Can you work these out from the model? Positions are in its coordinate system, mm. Give positions to 0.01 mm unless a question says otherwise; leave off trailing zeros. Order: outer loops, then holes, each group sorted by start corner. A loop starts at its lowest first (then second) coordinate and runs counter-clockwise, first axis right, second up. Notation, with made-up numbers: (0, 9.5) - (56, 9.5) arc R24 ccw to (56, 29.5) - close; hole circle Ø8 at (-24, -14.75). An arc over 180 degrees is marked (long way). Use one line per item in the form item = value. Start each with the question number.
1) Suppose I cut it at D-D, the plane z = -6. Write out the boundary of the cut face in (x, y), and give its area (3 significant figures).
2) For pin 1 (1.5 mm diameter, centred on x = 0.5, z = -2.5, fed in from +Y), with a flat end and sliding along its axis, tell me the tip position at first contact or that it passes through.
3) Suppose I cut it at C-C, the plane y = 0.2. Write out the boundary of the cut face in (x, z), and give its area (3 significant figures).
4) We'd pull the mould along X, two halves only. Please class faces 1 (the flat face through (0, 0.787, -3)), 2 (the flat face through (0, 0.66, -4.7)), 3 (the flat face through (-3.5, 0.4, -6.9)), 4 (the flat face through (3.5, 0.4, -6.9)): released by +X, released by -X, zero draft, split by the parting line, or undercut.
5) Please list where these lines run through material, in increasing order: probe 1 along X at (y, z) = (0.75, -5.25); probe 2 along Y at (x, z) = (-1.75, -2); probe 3 along Z at (x, y) = (0.75, 0.7).
6) Suppose I cut it at B-B, the plane z = -14.5. Write out the boundary of the cut face in (x, y), and give its area (3 significant figures).
```python
from build123d import *

# Parameters (mm, degrees)
SKETCH1_W           = 7
SKETCH1_H           = 11.4
BOSS_EXTRUDE1_DEPTH = 0.6604
BOSS_EXTRUDE2_DEPTH = 7
SKETCH4_R           = 1.07
SKETCH4_W           = 0.625641059
SKETCH4_H           = 1.254110087
BOSS_EXTRUDE3_DEPTH = 0.127
SKETCH5_R           = 0.1
BOSS_EXTRUDE4_DEPTH = 10


with BuildPart() as part:
    # Sketch1 → Boss-Extrude1 (new body)
    with BuildSketch(Plane(origin=(0, 0, 0), x_dir=(1, 0, 0), z_dir=(0, 1, 0))):
        with Locations((0, 5.7)):
            Rectangle(SKETCH1_W, SKETCH1_H)
    extrude(amount=BOSS_EXTRUDE1_DEPTH)

    # Sketch3 → Boss-Extrude2 (add)
    with BuildSketch(Plane.ZY.offset(3.5)):
        with BuildLine():
            Line((-11.4, 0.6604), (-11.4, 1.2))
            ThreePointArc((-11.4, 1.2), (-10.260013654, 1.483539887), (-9.25, 0.883676442))
            Line((-9.25, 0.883676442), (-9.25, 0.6604))
            Line((-9.25, 0.6604), (-11.4, 0.6604))
        make_face()
    extrude(amount=-BOSS_EXTRUDE2_DEPTH)

    # Sketch4 → Boss-Extrude3 (add)
    with BuildSketch(Plane(origin=(0, 0.6604, 0), x_dir=(1, 0, 0), z_dir=(0, 1, 0))):
        with Locations(Location((0, 3.4, 0), (0, 0, 270))):
            Circle(SKETCH4_R)
        with Locations((0.312820529, 5.772944956)):
            Rectangle(SKETCH4_W, SKETCH4_H)
        with BuildLine():
            Line((-0.625641059, 4.901538541), (-0.691025641, 5.058461538))
            ThreePointArc((-0.691025641, 5.058461538), (0, 1.603333333), (0.691025641, 5.058461538))
            Line((0.691025641, 5.058461538), (0.625641059, 4.901538541))
            ThreePointArc((0.625641059, 4.901538541), (0, 1.773333247), (-0.625641059, 4.901538541))
        make_face()
        with BuildLine():
            Line((0.905128238, 5.572307772), (0.970512821, 5.729230769))
            ThreePointArc((0.970512821, 5.729230769), (0, 0.876666667), (-0.970512821, 5.729230769))
            Line((-0.970512821, 5.729230769), (-0.905128238, 5.572307772))
            ThreePointArc((-0.905128238, 5.572307772), (0, 1.046666581), (0.905128238, 5.572307772))
        make_face()
        with BuildLine():
            Line((1.184615418, 6.243077002), (1.25, 6.4))
            ThreePointArc((1.25, 6.4), (0, 0.15), (-1.25, 6.4))
            Line((-1.25, 6.4), (-1.184615418, 6.243077002))
            ThreePointArc((-1.184615418, 6.243077002), (0, 0.319999914), (1.184615418, 6.243077002))
        make_face()
    extrude(amount=BOSS_EXTRUDE3_DEPTH)

    # Sketch5 → Boss-Extrude4 (add)
    with BuildSketch(Plane(origin=(0, 0, -11.4), x_dir=(-1, 0, 0), z_dir=(0, 0, -1))):
        with Locations(Location((-2.5, 0.7604, 0), (0, 0, 180))):
            Circle(SKETCH5_R)
        with Locations(Location((-1.5, 0.7604, 0), (0, 0, 180))):
            Circle(SKETCH5_R)
        with Locations(Location((-0.5, 0.7604, 0), (0, 0, 180))):
            Circle(SKETCH5_R)
        with Locations(Location((0.5, 0.7604, 0), (0, 0, 180))):
            Circle(SKETCH5_R)
        with Locations(Location((1.5, 0.7604, 0), (0, 0, 180))):
            Circle(SKETCH5_R)
        with Locations(Location((2.5, 0.7604, 0), (0, 0, 180))):
            Circle(SKETCH5_R)
    extrude(amount=BOSS_EXTRUDE4_DEPTH)


solid = part.part
```
Result sheet:
q1.outline = (-3.5, 0) - (3.5, 0) - (3.5, 0.66) - (1.95, 0.66) - (1.95, 0.79) - (1.65, 0.79) - (1.65, 0.66) - (0.63, 0.66) - (0.63, 0.79) - (0, 0.79) - (0, 0.66) - (-1.65, 0.66) - (-1.65, 0.79) - (-1.95, 0.79) - (-1.95, 0.66) - (-3.5, 0.66) - close
q1.area = 4.78 mm²
q2.pin_1 = 0.79
q3.outline = (-3.5, -11.4) - (3.5, -11.4) - (3.5, 0) - (-3.5, 0) - close
q3.area = 79.8 mm²
q4.face_1 = zero draft
q4.face_2 = undercut
q4.face_3 = released by -X
q4.face_4 = released by +X
q5.probe_1 = -2.67 to -2.46, -1.72 to -1.45, 0 to 0.63, 1.45 to 1.72, 2.46 to 2.67
q5.probe_2 = 0 to 0.66
q5.probe_3 = -11.4 to -9.25, -5.03 to -4.84, -4.16 to -2.64, -1.96 to -1.77, -1.17 to -0.99, -0.41 to -0.24
q6.outline = circle Ø0.2 at (-2.5, 0.76); circle Ø0.2 at (-1.5, 0.76); circle Ø0.2 at (-0.5, 0.76); circle Ø0.2 at (0.5, 0.76); circle Ø0.2 at (1.5, 0.76); circle Ø0.2 at (2.5, 0.76)
q6.area = 0.188 mm²
